from build123d import *

# Parameters (mm, degrees)
F0_R      = 10.66798
F1_DEPTH  = 1.5
F2_W      = 7.62
F2_H      = 15.24
F3_DEPTH  = 2.31
F4_W      = 4.445
F4_H      = 12.065
F5_DEPTH  = 10.16
F6_R      = 1.905
F7_DEPTH  = 13.971
F8_R      = 1.905
F9_DEPTH  = 3.81
F10_R     = 1.19378
F11_DEPTH = 1.501


with BuildPart() as f1:
    # F0 (on Top) → F1 (new body)
    with BuildSketch(Plane.XY):
        Circle(F0_R)
    extrude(amount=F1_DEPTH)

    # F2 (on face) → F3 (join)
    with BuildSketch(Plane.XY.offset(1.5)):
        Rectangle(F2_W, F2_H)
    extrude(amount=F3_DEPTH)

    # F4 (on face) → F5 (join)
    with BuildSketch(Plane.XY.offset(3.81)):
        Rectangle(F4_W, F4_H)
    extrude(amount=F5_DEPTH)

    # F6 (on face) → F7 (cut, through all)
    with BuildSketch(Plane.XY.offset(13.97)):
        Circle(F6_R)
    extrude(amount=-F7_DEPTH, mode=Mode.SUBTRACT)

    # F8 (on face) → F9 (cut)
    with BuildSketch(Plane(origin=(0, 0, 0), x_dir=(1, 0, 0), z_dir=(0, 0, -1))):
        Polygon((4.064, 2.346351), (0, 4.692703), (-4.064, 2.346351), (-4.064, -2.346351), (0, -4.692703), (4.064, -2.346351), align=None)
        Circle(F8_R, mode=Mode.SUBTRACT)
    extrude(amount=-F9_DEPTH, mode=Mode.SUBTRACT)

    # F10 (on face) → F11 (cut, through all)
    with BuildSketch(Plane.XY.offset(1.5)):
        with Locations((-6, 0)):
            Circle(F10_R)
        with Locations((6, 0)):
            Circle(F10_R)
    extrude(amount=-F11_DEPTH, mode=Mode.SUBTRACT)


solid = f1.part
Work out the finished part from the listing and answer in its coordinate system (mm). A direction names the side the tool comes from. Round coordinates to 2 decimals unless told otherwise and drop trailing zeros. Write each loop counter-clockwise with the first axis right and the second up, starting at its lowest first coordinate (ties: lowest second). Pieces come first, ordered by that corner, then holes.
1) Given pin 1 Ø1.2 at (y, z) = (5, 2.5) entering from -X; pin 2 Ø1 at (x, z) = (2, 5) entering from +Y; pin 3 Ø1.5 at (x, z) = (1, 2) entering from +Y, each flat-ended and moving along its own axis, determine where each tip first touches the part or whether it passes through.
2) A cutting plane is placed at A-A (y = 0). Give the number of separate pieces and of enclosed holes in the cut face, plus the area to 3 significant figures.
3) The mould has two halves that part along Y. Classify faces 1 (the flat face through (0, 7.62, 3)), 2 (the cylindrical face through (-0.41, -1.86, 8.96)), 3 (the cylindrical face through (-10.658, 0.469, 0.74)): pulls with the +Y half, pulls with the -Y half, needs draft (parallel to the pull), parting line crosses it, or undercut.
4) A cutting plane is placed at D-D (y = -3). Give the vertices of the cut face in (x, z).
5) Straight lines are drawn through the part: line 1 (X direction, y = 0, z = 6.75) (1 decimal); line 2 (Z direction, x = -7.75, y = -1.5); line 3 (Z direction, x = 2, y = 1). For each, find the intervals that lie inside material, in ascending order.
6) A cutting plane is placed at B-B (z = 11). Give the vertices of the cut face in (x, y) (1 decimal), plus the area to 3 significant figures.
7) A tool of negligible diameter and unlimited length cuts with its end or side. For faces 4 (the flat face through (-2.222, 0, 9)), 5 (the flat face through (0, -7.62, 3)), 6 (the flat face through (0.5, 2, 3.81)), from which of +Z, -Z, +X, -X, +Y, -Y can it reach the whole face along a straight path? Write none if from no direction.
8) A cutting plane is placed at C-C (x = 6). Give the vertices of the cut face in (y, z), plus the area to 3 significant figures.
Completed:
1. pin 1: stops at x = -3.81
1. pin 2: stops at y = 6.03
1. pin 3: stops at y = 10.66
2. separate pieces: 6
2. enclosed holes: 0
2. area: 19.1 mm2
3. face 1: pulls with the +Y half
3. face 2: undercut
3. face 3: parting line crosses it
4. outline: (-10.24, 0) - (-2.93, 0) - (-2.93, 3.81) - (-3.81, 3.81) - (-3.81, 1.5) - (-10.24, 1.5) - close; (-2.22, 3.81) - (2.22, 3.81) - (2.22, 13.97) - (-2.22, 13.97) - close; (2.93, 0) - (10.24, 0) - (10.24, 1.5) - (3.81, 1.5) - (3.81, 3.81) - (2.93, 3.81) - close
5. line 1: x = -2.2 to -1.9, 1.9 to 2.2
5. line 2: z = 0 to 1.5
5. line 3: z = 3.81 to 13.97
6. outline: (-2.2, -6) - (2.2, -6) - (2.2, 6) - (-2.2, 6) - close; hole circle Ø3.8 at (0, 0)
6. area: 42.2 mm2
7. face 4: +Z, -X, +Y, -Y
7. face 5: +Z, +X, -X, -Y
7. face 6: -Z
8. outline: (-8.82, 0) - (-1.19, 0) - (-1.19, 1.5) - (-8.82, 1.5) - close; (1.19, 0) - (8.82, 0) - (8.82, 1.5) - (1.19, 1.5) - close
8. area: 22.9 mm2
